Autodesk Inventor part; units mm, degrees
ref_plane "YZ Plane" through (0, 0, 0) normal (1, 0, 0) x (0, 1, 0)
ref_plane "XZ Plane" through (0, 0, 0) normal (0, 1, 0) x (-1, 0, 0)
ref_plane "XY Plane" through (0, 0, 0) normal (0, 0, 1) x (1, 0, 0)
sketch "Sketch1" plane through (0, 0, 0) normal (1, 0, 0) x (0, 1, 0)
  arc A0 (7.1618, 41.4339) -> (-20.3375, 41.4339) centre (-6.5878, 41.4339) ccw
  arc A1 (-20.3375, -36.0661) -> (7.1618, -36.0661) centre (-6.5878, -36.0661) ccw
  line L0 (7.1618, 41.4339) -> (7.1618, -36.0661)
  line L1 (-20.3375, -36.0661) -> (-20.3375, 41.4339)
  line L2 (8.9018, -36.0661) -> (8.9018, 41.4339)
  arc A2 (8.9018, 41.4339) -> (-22.0775, 41.4339) centre (-6.5878, 41.4339) ccw
  line L3 (-22.0775, 41.4339) -> (-22.0775, -36.0661)
  arc A3 (-22.0775, -36.0661) -> (8.9018, -36.0661) centre (-6.5878, -36.0661) ccw
  point P0 (0, 0)
  dimension "d0" = 27.4993
  dimension "d1" = 27.4993
  dimension "d2" = 77.5
  dimension "d3" = 0
  dimension "d4" = 1.74
extrude "Extrusion1" add sketch "Sketch1" along normal blind 9
equation "\"d1\" = d0"
properties part number "49T belt from gobuilda"
The listing builds one solid part. Answer for the finished solid, in the listing's coordinates (mm). A direction names the side the tool comes from. Coordinates: 2 decimals unless noted, no trailing zeros. Loops run counter-clockwise (first coordinate to the right, second up) from the corner with the lowest first, then second, coordinate; pieces in that order, holes last. Notation, with made-up numbers: (52, -2.5) - (81, -2.5) arc R19 cw to (81, 11.5) - close; hole circle Ø3 at (78.25, -14.75). An arc over 180 degrees is marked (long way). Use a Markdown table: item, result. Add a question column.
1) For faces 4 (the cylindrical face through (4.44, -6.89, 55.18)), 5 (the flat face through (0, -21.6, 7)), determine the directions among +Z, -Z, +X, -X, +Y, -Y from which every point of the face is accessible in a straight line to the end or side of a thin tool.
2) The part is cut by section A-A, the plane z = 36.5. Give the vertices of the cut face in (x, y), and give its area (3 significant figures).
3) Given pin 1 (1 mm diameter, centred on x = 6, z = 43.5, fed in from +Y); pin 2 (5 mm diameter, centred on x = 7, y = -3, fed in from -Z); pin 3 (2 mm diameter, centred on x = 6.5, y = -10, fed in from +Z), each flat-ended and moving along its own axis, determine where each tip first touches the part or whether it passes through.
4) Find the intervals of material crossed by line 1 (Y direction, x = 6.5, z = 30); line 2 (Y direction, x = 1, z = 42); line 3 (Z direction, x = 7.25, y = -5), in increasing order.
5) The part is cut by section B-B, the plane x = 3.75. Give the vertices of the cut face in (y, z).
6) The mould has two halves that part along Y. Classify faces 1 (the flat face through (4, -22.078, 3)), 2 (the flat face through (4, -20.338, 2)), 3 (the cylindrical face through (4.44, -6.93, 56.92)): released by +Y, released by -Y, zero draft, split by the parting line, or undercut.
7) The part is cut by section C-C, the plane y = -4. Give the vertices of the cut face in (x, z).
Here are the results:
| question | item | result |
|---|---|---|
| 1 | face 4 | +X, -X |
| 1 | face 5 | +Z, -Z, -X, +Y, -Y |
| 2 | outline | (0, -22.08) - (9, -22.08) - (9, -20.34) - (0, -20.34) - close; (0, 7.16) - (9, 7.16) - (9, 8.9) - (0, 8.9) - close |
| 2 | area | 31.3 mm^2 |
| 3 | pin 1 | stops at y = 8.82 |
| 3 | pin 2 | stops at z = -51.52 |
| 3 | pin 3 | stops at z = 56.73 |
| 4 | line 1 | y = -22.08 to -20.34, 7.16 to 8.9 |
| 4 | line 2 | y = -22.07 to -20.33, 7.15 to 8.89 |
| 4 | line 3 | z = -51.47 to -49.72, 55.09 to 56.84 |
| 5 | outline | (-22.08, -36.07) arc R15.49 ccw to (8.9, -36.07) - (8.9, 41.43) arc R15.49 ccw to (-22.08, 41.43) - close; hole (-20.34, -36.07) arc R13.75 ccw to (7.16, -36.07) - (7.16, 41.43) arc R13.75 ccw to (-20.34, 41.43) - close |
| 6 | face 1 | released by -Y |
| 6 | face 2 | undercut |
| 6 | face 3 | split by the parting line |
| 7 | outline | (0, -51.34) - (9, -51.34) - (9, -49.57) - (0, -49.57) - close; (0, 54.94) - (9, 54.94) - (9, 56.71) - (0, 56.71) - close |
